Could you check a few things on this drawing? It's one solid part, dimensions in mm from its lowest x, y, z. A direction names the side the tool comes from. Round coordinates to 2 decimals unless told otherwise and drop trailing zeros. Loops run counter-clockwise (first coordinate to the right, second up) from the corner with the lowest first, then second, coordinate; pieces in that order, holes last. Notation, with made-up numbers: M -29,89.5 L 12,89.5 A27 ccw 12,121.5 Z; hole C -11,-6 d2. An arc over 180 degrees is marked long. Write item = value, one per line. Start each with the question number.
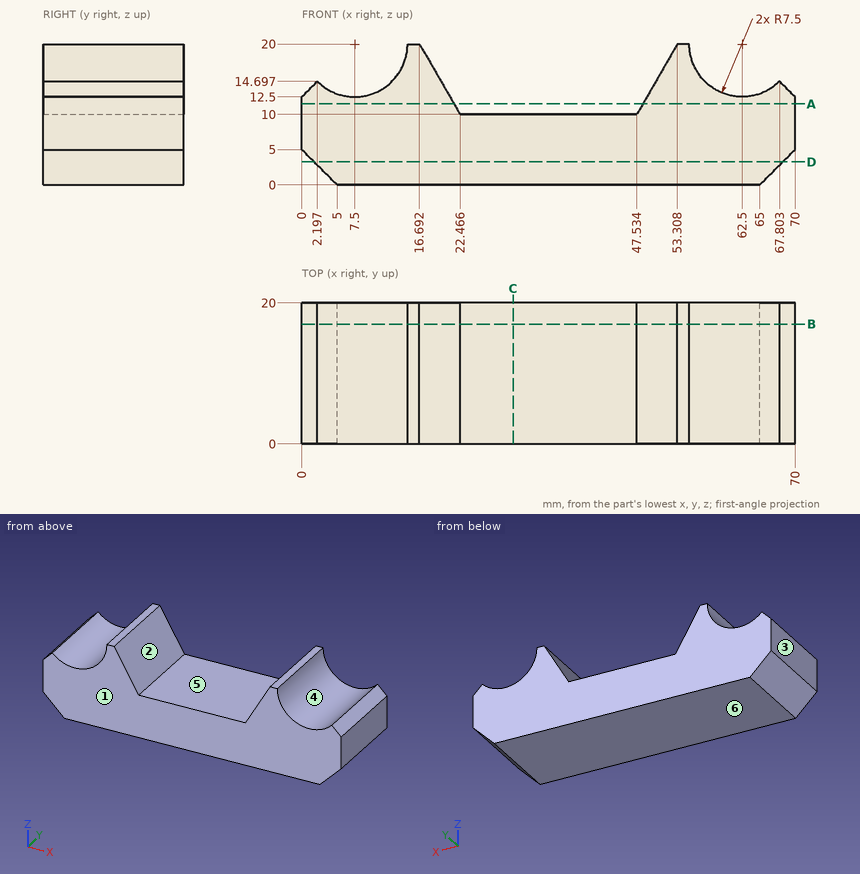
Item 1: Please list where these lines run through material, in increasing order: line 1 (X direction, y = 13.5, z = 13.5) (1 decimal); line 2 (Z direction, x = 23.5, y = 13); line 3 (X direction, y = 9.5, z = 14.75) (1 decimal). Write a range as [from, to].
Item 2: For the marked faces 5 and 6, which set-ups out of +Z, -Z, +X, -X, +Y, -Y let a thin tool reach every point of the face, with its end or its side?
Item 3: I want a section at A-A, the plane z = 11.5. List the corners of the cut face in (x, y) for me.
Item 4: I want a section at D-D, the plane z = 3.25. List the corners of the cut face in (x, y) for me.
Item 5: We'd pull the mould along X, two halves only. Please class the marked faces 1, 2, 3 and 4: released by +X, released by -X, zero draft, split by the parting line, or undercut.
Item 6: Will these pins go through, and if not, where does the flat tip stop? pin 1 Ø4 at (y, z) = (8.5, 17) entering from -X; pin 2 Ø10 at (x, y) = (40.5, 12) entering from +Z; pin 3 Ø10 at (x, y) = (44.5, 5.5) entering from +Z (1 decimal).
Item 7: I want a section at C-C, the plane x = 30. List the corners of the cut face in (y, z) for me.
Item 8: I want a section at B-B, the plane y = 17. List the corners of the cut face in (x, z) for me, then the cut area to 3 significant figures.
Worked out:
q1.line_1 = [1, 3.8], [11.2, 20.4], [49.6, 58.8], [66.2, 69]
q1.line_2 = [0, 10]
q1.line_3 = [12.9, 19.7], [50.3, 57.1]
q2.face_5 = +Z, +Y, -Y
q2.face_6 = -Z, +X, -X, +Y, -Y
q3.outline = M 0,0 L 21.6,0 L 21.6,20 L 0,20 Z; M 48.4,0 L 70,0 L 70,20 L 48.4,20 Z
q4.outline = M 1.75,0 L 68.25,0 L 68.25,20 L 1.75,20 Z
q5.face_1 = zero draft
q5.face_2 = undercut
q5.face_3 = released by -X
q5.face_4 = undercut
q6.pin_1 = 13.09
q6.pin_2 = 10
q6.pin_3 = 13.4
q7.outline = M 0,0 L 20,0 L 20,10 L 0,10 Z
q8.outline = M 0,5 L 5,0 L 65,0 L 70,5 L 70,12.5 L 67.8,14.7 A7.5 cw 55,20 L 53.31,20 L 47.53,10 L 22.47,10 L 16.69,20 L 15,20 A7.5 cw 2.2,14.7 L 0,12.5 Z
q8.area = 878 mm2
